```python
from build123d import *

# Parameters (mm, degrees)
SKETCH1_W               = 300
SKETCH1_H               = 150
SKETCH1_W_2             = 220
SKETCH1_H_2             = 50
BOSS_EXTRUDE2_DEPTH     = 15
SKETCH2_W               = 220
SKETCH2_H               = 18
BOSS_EXTRUDE3_DEPTH     = 3
MIRROR2_COPY_1_SKETCH_W = 220
MIRROR2_COPY_1_SKETCH_H = 18
MIRROR2_COPY_1_DEPTH    = 3
SKETCH3_W               = 220
SKETCH3_H               = 14
BOSS_EXTRUDE4_DEPTH     = 2
SKETCH5_R               = 8.5
CUT_EXTRUDE2_DEPTH      = 5
SKETCH6_W               = 50
SKETCH6_H               = 50
SKETCH6_R               = 2.5
BOSS_EXTRUDE5_DEPTH     = 40
FILLET3_R               = 5


with BuildPart() as part:
    # Sketch1 → Boss-Extrude2 (new body, symmetric)
    with BuildSketch(Plane.XY):
        Rectangle(SKETCH1_W, SKETCH1_H)
        Rectangle(SKETCH1_W_2, SKETCH1_H_2, mode=Mode.SUBTRACT)
    extrude(amount=BOSS_EXTRUDE2_DEPTH, both=True)

    # Sketch2 → Boss-Extrude3 (add)
    with BuildSketch(Plane.XY.offset(15)):
        with Locations((0, 16)):
            Rectangle(SKETCH2_W, SKETCH2_H)
    boss_extrude3 = extrude(amount=-BOSS_EXTRUDE3_DEPTH)

    # Mirror1: Boss-Extrude3 across plane
    add(boss_extrude3.mirror(Plane.XY))

    # Mirror2: Boss-Extrude3 across plane
    add(boss_extrude3.mirror(Plane.ZX))

    # Mirror2 copy 1 sketch → Mirror2 copy 1 (add)
    with BuildSketch(Plane(origin=(0, 0, -15), x_dir=(1, 0, 0), z_dir=(0, 0, -1))):
        with Locations((0, 16)):
            Rectangle(MIRROR2_COPY_1_SKETCH_W, MIRROR2_COPY_1_SKETCH_H)
    extrude(amount=-MIRROR2_COPY_1_DEPTH)

    # Sketch3 → Boss-Extrude4 (add)
    with BuildSketch(Plane(origin=(0, 0, -15), x_dir=(-1, 0, 0), z_dir=(0, 0, -1))):
        Rectangle(SKETCH3_W, SKETCH3_H)
    extrude(amount=-BOSS_EXTRUDE4_DEPTH)

    # Sketch5 → Cut-Extrude2 (cut)
    with BuildSketch(Plane(origin=(0, 75, 0), x_dir=(1, 0, 0), z_dir=(0, 1, 0))):
        with Locations((-100, 0)):
            Circle(SKETCH5_R)
        with Locations((100, 0)):
            Circle(SKETCH5_R)
    cut_extrude2 = extrude(amount=-CUT_EXTRUDE2_DEPTH, mode=Mode.SUBTRACT)

    # Mirror3: Cut-Extrude2 across plane
    add(cut_extrude2.mirror(Plane.ZX), mode=Mode.SUBTRACT)

    # Sketch6 → Boss-Extrude5 (add)
    with BuildSketch(Plane.XY.offset(15)):
        with Locations((95, 0)):
            Rectangle(SKETCH6_W, SKETCH6_H)
        with Locations((95, 0)):
            Circle(SKETCH6_R, mode=Mode.SUBTRACT)
    extrude(amount=BOSS_EXTRUDE5_DEPTH)

    # Fillet3
    fillet3_edges = [part.edges().sort_by_distance(p)[0] for p in [
        (70, -16, 15),
        (120, 0, 55),
        (95, 25, 55),
        (70, 0, 55),
        (95, -25, 55),
        (120, 0, 15),
        (120, -25, 35),
        (95, 25, 15),
        (120, 25, 35),
        (70, 16, 15),
        (70, 25, 35),
        (95, -25, 15),
        (70, -25, 35),
    ]]
    fillet(fillet3_edges, radius=FILLET3_R)


solid = part.part
```
Geometry check sheet. Reference: the model listing, model coordinates, mm. A direction names the side the tool comes from. Round coordinates to 2 decimals unless told otherwise and drop trailing zeros. Order: outer loops, then holes, each group sorted by start corner. A loop starts at its lowest first (then second) coordinate and runs counter-clockwise, first axis right, second up. Notation, with made-up numbers: M 25,34.25 L 54,34.25 A23 cw 54,63.25 Z; hole C 62.5,-20 d4. An arc over 180 degrees is marked long. Write item = value, one per line.
Q1. Set-up check for faces 4 (the flat face through (-2, 25, 0)), 5 (the flat face through (95, -25, 35)), 6 (the cylindrical face through (91.51, 72.54, -0.37)), 7 (the flat face through (120, 0, 35)): record each of +Z, -Z, +X, -X, +Y, -Y from which the full face is reachable in a straight line by a thin tool's end or side.
Answer block:
face_4 = none
face_5 = +Z, +X, -X, -Y
face_6 = +Y
face_7 = +Z, +X, +Y, -Y
Q2. Section check A-A (z = 0). Enter the section's corners in (x, y).
Answer block:
outline = M -150,-75 L -108.5,-75 L -108.5,-70 L -91.5,-70 L -91.5,-75 L 91.5,-75 L 91.5,-70 L 108.5,-70 L 108.5,-75 L 150,-75 L 150,75 L 108.5,75 L 108.5,70 L 91.5,70 L 91.5,75 L -91.5,75 L -91.5,70 L -108.5,70 L -108.5,75 L -150,75 Z; hole M -110,-25 L 110,-25 L 110,25 L -110,25 Z
Q3. Section check B-B (y = -12). Enter the section's corners in (x, z), plus the area to 3 significant figures.
Answer block:
outline = M -150,-15 L 150,-15 L 150,15 L 125,15 A5 cw 120,20 L 120,50 A5 ccw 115,55 L 75,55 A5 ccw 70,50 L 70,20 A5 cw 65,15 L -150,15 Z; hole M -110,-12 L 110,-12 L 110,12 L -110,12 Z
area = 5,720 mm^2
Q4. Depth check by flat-ended pin: pin 1 Ø24 at (x, z) = (87.5, 31.5) entering from +Y; pin 2 Ø20 at (x, y) = (-8, -13) entering from +Z; pin 3 Ø15.5 at (x, z) = (-100, 0) entering from -Y; pin 4 Ø6 at (x, z) = (42.5, 19) entering from +Y. Enter the tip coordinate at first touch or a pass-through.
Answer block:
pin_1 = 25.03
pin_2 = 15
pin_3 = -70
pin_4 = through
Q5. Section check C-C (x = -29). Enter the section's corners in (y, z).
Answer block:
outline = M -75,-15 L 75,-15 L 75,15 L 7,15 L 7,12 L 25,12 L 25,-12 L 7,-12 L 7,-13 L -7,-13 L -7,-12 L -25,-12 L -25,12 L -7,12 L -7,15 L -75,15 Z
Q6. Release check for a two-part mould opening along X. For faces 1 (the flat face through (-2, 16, -12)), 2 (the flat face through (70, 0, 32)), 3 (the flat face through (-2, -75, 0)) record: released by +X, released by -X, zero draft, split by the parting line, or undercut.
Answer block:
face_1 = undercut
face_2 = released by -X
face_3 = zero draft
Q7. Section check D-D (z = 37.5). Enter the section's corners in (x, y).
Answer block:
outline = M 70,-20 A5 ccw 75,-25 L 115,-25 A5 ccw 120,-20 L 120,20 A5 ccw 115,25 L 75,25 A5 ccw 70,20 Z; hole C 95,0 d5
Q8. Scan lines: line 1 (X direction, y = 72.2, z = 0); line 2 (Z direction, x = 100, y = 71.9); line 3 (Y direction, x = 95, z = 23). Record each from-to range of solid material in increasing order.
Answer block:
line_1 = -150 to -108.5, -91.5 to 91.5, 108.5 to 150
line_2 = -15 to -8.5, 8.5 to 15
line_3 = -25 to -2.5, 2.5 to 25
